```python
from build123d import *

# Parameters (mm, degrees)
SKETCH_1_W          = 199
SKETCH_1_H          = 99
EXTRUDE_1_DEPTH     = 9
SKETCH_2_W          = 199
SKETCH_2_H          = 2
EXTRUDE_2_DEPTH     = 41
SKETCH_4_W          = 199
SKETCH_4_H          = 2
EXTRUDE_3_DEPTH     = 41
SKETCH_5_W          = 184
SKETCH_5_H          = 95
EXTRUDE_4_DEPTH     = 41
SKETCH_6_R          = 2
CUT_EXTRUDE_2_DEPTH = 10
CUT_EXTRUDE_3_DEPTH = 10
SKETCH_10_R         = 2
CUT_EXTRUDE_4_DEPTH = 158.091394395
SKETCH_11_R         = 1.5
CUT_EXTRUDE_5_DEPTH = 6


with BuildPart() as part:
    # 草图1 → 凸台-拉伸1 (new body)
    with BuildSketch(Plane(origin=(0, 0, 0), x_dir=(1, 0, 0), z_dir=(0, 1, 0))):
        with Locations((11.750645809, -1.511939619)):
            Rectangle(SKETCH_1_W, SKETCH_1_H)
    extrude(amount=EXTRUDE_1_DEPTH)

    # 草图2 → 凸台-拉伸2 (add)
    with BuildSketch(Plane(origin=(0, 9, 0), x_dir=(1, 0, 0), z_dir=(0, 1, 0))):
        with Locations((11.750645809, -50.011939619)):
            Rectangle(SKETCH_2_W, SKETCH_2_H)
    extrude(amount=EXTRUDE_2_DEPTH)

    # 草图4 → 凸台-拉伸3 (add)
    with BuildSketch(Plane(origin=(0, 9, 0), x_dir=(1, 0, 0), z_dir=(0, 1, 0))):
        with Locations((11.750645809, 46.988060381)):
            Rectangle(SKETCH_4_W, SKETCH_4_H)
    extrude(amount=EXTRUDE_3_DEPTH)

    # 草图5 → 凸台-拉伸4 (add)
    with BuildSketch(Plane(origin=(0, 9, 0), x_dir=(1, 0, 0), z_dir=(0, 1, 0))):
        with Locations((19.250645809, -1.511939619)):
            Rectangle(SKETCH_5_W, SKETCH_5_H)
    extrude(amount=EXTRUDE_4_DEPTH)

    # 草图6 → 切除-拉伸2 (cut)
    with BuildSketch(Plane.XY.offset(51.011939619)):
        with Locations((87.250645809, 37.5)):
            Circle(SKETCH_6_R)
        with Locations((87.250645809, 12.5)):
            Circle(SKETCH_6_R)
        with Locations((-62.749354191, 12.5)):
            Circle(SKETCH_6_R)
        with Locations((-62.749354191, 37.5)):
            Circle(SKETCH_6_R)
    extrude(amount=-CUT_EXTRUDE_2_DEPTH, mode=Mode.SUBTRACT)

    # 草图8 → 切除-拉伸3 (cut)
    with BuildSketch(Plane.XY.offset(51.011939619)):
        with BuildLine():
            ThreePointArc((-77.764739213, 37.714285714), (-79.249354191, 39), (-80.733969169, 37.714285714))
            ThreePointArc((-80.733969169, 37.714285714), (-83.249345598, 34.00829113), (-80.749354191, 30.291900756))
            Line((-80.749354191, 30.291900756), (-80.749354191, 20.5))
            ThreePointArc((-80.749354191, 20.5), (-79.249354191, 19), (-77.749354191, 20.5))
            Line((-77.749354191, 20.5), (-77.749354191, 30.291900756))
            ThreePointArc((-77.749354191, 30.291900756), (-75.249362784, 34.00829113), (-77.764739213, 37.714285714))
        make_face()
    extrude(amount=-CUT_EXTRUDE_3_DEPTH, mode=Mode.SUBTRACT)

    # 草图10 → 切除-拉伸4 (cut, through all)
    with BuildSketch(Plane(origin=(0, 0, -47.988060381), x_dir=(-1, 0, 0), z_dir=(0, 0, -1))):
        with Locations(Location((62.749354191, 12.5, 0), (0, 0, 180))):
            Circle(SKETCH_10_R)
        with Locations(Location((-87.250645809, 12.5, 0), (0, 0, 180))):
            Circle(SKETCH_10_R)
    extrude(amount=-CUT_EXTRUDE_4_DEPTH, mode=Mode.SUBTRACT)

    # 草图11 → 切除-拉伸5 (cut)
    with BuildSketch(Plane(origin=(0, 0, 0), x_dir=(-1, 0, 0), z_dir=(0, -1, 0))):
        with Locations(Location((72.749354191, 23.488060381, 0), (0, 0, 90))):
            Circle(SKETCH_11_R)
        with Locations(Location((72.749354191, -26.511939619, 0), (0, 0, 90))):
            Circle(SKETCH_11_R)
        with Locations(Location((-77.250645809, 23.488060381, 0), (0, 0, 90))):
            Circle(SKETCH_11_R)
        with Locations(Location((-77.250645809, -26.511939619, 0), (0, 0, 90))):
            Circle(SKETCH_11_R)
    extrude(amount=-CUT_EXTRUDE_5_DEPTH, mode=Mode.SUBTRACT)


solid = part.part
```
The listing builds one solid part. Answer for the finished solid, in the listing's coordinates (mm). A direction names the side the tool comes from. Give positions to 0.01 mm unless a question says otherwise; leave off trailing zeros. Loops run counter-clockwise (first coordinate to the right, second up) from the corner with the lowest first, then second, coordinate; pieces in that order, holes last. Notation, with made-up numbers: M 80,12.5 L 117,12.5 A23 cw 117,33.5 Z; hole C 41.5,-3.75 d11. An arc over 180 degrees is marked long. One line per item, written item: value.
Q1. For faces 1 (the face through (-60.902, 36.734, 46.082)), 2 (the face through (-87.749, 8, 9)), 3 (the face through (-80, 29, -45.988)), determine the directions among +Z, -Z, +X, -X, +Y, -Y from which every point of the face is accessible in a straight line to the end or side of a thin tool.
Working result:
face 1: +Z
face 2: +Z, -Z, -X, +Y, -Y
face 3: -X, +Y
Q2. Determine the mould class of faces 4 (the face through (-80, 9, 1)), 5 (the face through (89.16, 13.1, 2.2)), 6 (the face through (87, 38, 41.012)), 7 (the face through (-82, 29, 49.012)) for opening direction Z: +Z half, -Z half, draft (parallel to the pull), parting line (faces both ways), or undercut.
Working result:
face 4: undercut
face 5: draft
face 6: +Z half
face 7: undercut
Q3. A cutting plane is placed at B-B on y = 12.5. Determine the outline of the cut face in (x, z), then the cut area to 3 significant figures.
Working result:
outline: M -87.75,-47.99 L -64.75,-47.99 L -64.75,51.01 L -87.75,51.01 L -87.75,49.01 L -72.75,49.01 L -72.75,-45.99 L -87.75,-45.99 Z; M -60.75,-47.99 L 85.25,-47.99 L 85.25,51.01 L -60.75,51.01 Z; M 89.25,-47.99 L 111.25,-47.99 L 111.25,51.01 L 89.25,51.01 Z
area: 17,500 mm^2
Q4. Find the intervals of material crossed by line 1 (X direction, y = 12.5, z = -5); line 2 (Z direction, x = -74, y = 16); line 3 (X direction, y = 43, z = 30.5), in increasing order. Write a range as from..to.
Working result:
line 1: x = -72.75..-64.75, -60.75..85.25, 89.25..111.25
line 2: z = -47.99..-45.99, 49.01..51.01
line 3: x = -72.75..111.25
Q5. A cutting plane is placed at C-C on y = 42. Determine the outline of the cut face in (x, z), then the cut area to 3 significant figures.
Working result:
outline: M -87.75,-47.99 L 111.25,-47.99 L 111.25,51.01 L -87.75,51.01 L -87.75,49.01 L -72.75,49.01 L -72.75,-45.99 L -87.75,-45.99 Z
area: 18,300 mm^2
Q6. Flat-ended cylindrical pins translate along their axes: P1, Ø5, axis at x = -17.5, z = -19, coming from the -Y side; P2, Ø3, axis at x = 87.25, y = 37.5, coming from the +Z side; P3, Ø4.5, axis at x = -78.5, z = -20, coming from the +Y side; P4, Ø1.5, axis at x = 77, z = -24, coming from the -Y side. Find the tip coordinate at first contact, or state that the pin passes through.
Working result:
P1: stops at y = 0
P2: stops at z = 41.01
P3: stops at y = 9
P4: stops at y = 6
Q7. A cutting plane is placed at A-A on z = 36. Determine the outline of the cut face in (x, y), then the cut area to 3 significant figures.
Working result:
outline: M -87.75,0 L 111.25,0 L 111.25,50 L -72.75,50 L -72.75,9 L -87.75,9 Z; hole C -62.75,12.5 d4; hole C 87.25,12.5 d4
area: 9,310 mm^2
